The listing builds one solid part. Answer for the finished solid, in the listing's coordinates (mm). Face numbers are marked on the shaded views. Round coordinates to 2 decimals unless told otherwise and drop trailing zeros. Write each loop counter-clockwise with the first axis right and the second up, starting at its lowest first coordinate (ties: lowest second). Pieces come first, ordered by that corner, then holes. Notation, with made-up numbers: M 15.25,-37 L 21.25,-37 A30 cw 21.25,0 Z; hole C 58.25,7.25 d10. An arc over 180 degrees is marked long. Write each question's results on one line, items separated by ' | '.
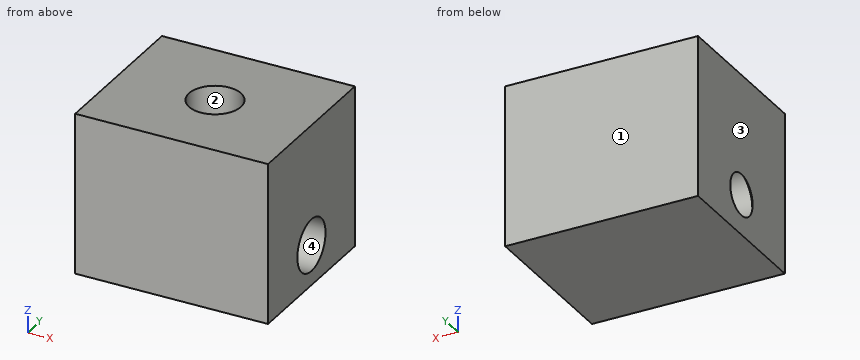
Autodesk Inventor part; units mm, degrees
ref_plane "YZ Plane" through (0, 0, 0) normal (1, 0, 0) x (0, 1, 0)
ref_plane "XZ Plane" through (0, 0, 0) normal (0, 1, 0) x (-1, 0, 0)
ref_plane "XY Plane" through (0, 0, 0) normal (0, 0, 1) x (1, 0, 0)
sketch "Skizze1" plane through (0, 0, 0) normal (0, 0, 1) x (1, 0, 0)
  line L0 (0, 0) -> (12, 0)
  line L1 (12, 0) -> (12, 10)
  line L2 (12, 10) -> (0, 10)
  line L3 (0, 10) -> (0, 0)
  dimension "d0" = 10
  dimension "d1" = 12
extrude "Extrusion1" add sketch "Skizze1" along normal blind 10
sketch "Skizze2" plane through (12, 0, 0) normal (1, 0, 0) x (0, 0, -1)
  line L0 (0, 0) -> (0, 10)
  line L1 (0, 10) -> (-10, 10)
  line L2 (-10, 0) -> (-10, 10)
  line L3 (0, 0) -> (-10, 0)
  line L4 (-10, 5) -> (0, 5) construction
  point P0 (-2.5, 5)
  dimension "d4" = 2.5
hole "Bohrung1" at (12, 5, 2.5) direction (-1, 0, 0) diameter 3.242 depth 11.8 tip angle 118
sketch "Skizze3" plane through (0, 0, 10) normal (0, 0, 1) x (1, 0, 0)
  line L0 (0, 0) -> (12, 0)
  line L1 (12, 0) -> (12, 10)
  line L2 (12, 10) -> (0, 10)
  line L3 (0, 10) -> (0, 0)
  line L4 (12, 6.621) -> (12, 3.379)
  line L5 (0.2, 3.379) -> (0.2, 6.621)
  line L6 (-2.4, 5) -> (14.4, 5)
  line L7 (6, 0) -> (6, 10) construction
  point P0 (6, 5)
  point P1 (6, 5)
hole "Bohrung2" at (6, 5, 10) direction (0, 0, -1) diameter 3.242 end up to surface
properties part number "Alu_Belt_tens_3" material "Aluminium 6061"
1) Find the intervals of material crossed by line 1 (X direction, y = 5, z = 7.5); line 2 (Y direction, x = 4.25, z = 2.5); line 3 (Z direction, x = 3.5, y = 5), in increasing order.
Return value:
line 1: 0 to 4.38, 7.62 to 12 | line 2: 0 to 3.38, 6.62 to 10 | line 3: 0 to 0.88, 4.12 to 10
2) The mould has two halves that part along Y. Classify the marked faces 1, 2, 3 and 4: +Y half, -Y half, draft (parallel to the pull), parting line (faces both ways), or undercut.
Return value:
face 1: +Y half | face 2: undercut | face 3: draft | face 4: undercut
3) Section B-B (x = 3) is taken. Determine the outline of the cut face in (y, z).
Return value:
outline: M 0,0 L 10,0 L 10,10 L 0,10 Z; hole C 5,2.5 d3.24
4) Section C-C (y = 5) is taken. Determine the outline of the cut face in (x, z).
Return value:
outline: M 0,0 L 12,0 L 12,0.88 L 0.2,0.88 L 0,1.21 Z; M 0,3.79 L 0.2,4.12 L 4.38,4.12 L 4.38,10 L 0,10 Z; M 7.62,4.12 L 12,4.12 L 12,10 L 7.62,10 Z
5) Section A-A (z = 4.5) is taken. Determine the outline of the cut face in (x, y), then the cut area to 3 significant figures.
Return value:
outline: M 0,0 L 12,0 L 12,10 L 0,10 Z; hole C 6,5 d3.24 | area: 112 mm²
6) Section D-D (x = 6) is taken. Determine the outline of the cut face in (y, z).
Return value:
outline: M 0,0 L 10,0 L 10,10 L 6.62,10 L 6.62,2.5 A1.62 cw 3.38,2.5 L 3.38,10 L 0,10 Z
